Geometry check sheet. Reference: the model listing, model coordinates, mm. Coordinates: 2 decimals unless noted, no trailing zeros. Write each loop counter-clockwise with the first axis right and the second up, starting at its lowest first coordinate (ties: lowest second). Pieces come first, ordered by that corner, then holes. Notation, with made-up numbers: (53.5, 89) -> (110.5, 89) arc R18 ccw to (110.5, 105) -> close; hole circle Ø11 at (30.25, -1). An arc over 180 degrees is marked (long way). Answer in a Markdown table with one row per item. Add a question column.
Q1. Section check C-C, the plane x = 18. Record the boundary of the cut face in (y, z).
Q2. Section check B-B, the plane x = 63. Record the boundary of the cut face in (y, z), and give its area (3 significant figures).
Q3. Section check A-A, the plane z = 0. Record the boundary of the cut face in (x, y).
Q4. Section check D-D, the plane y = 0.9. Record the boundary of the cut face in (x, z).
Q5. Gauge pin test, flat ends, axial feed: P1, Ø3, axis at x = -63.5, z = 23.5, coming from the +Y side; P2, Ø2.5, axis at x = -19, z = -2, coming from the -Y side. Record the tip position at first contact, or that the pin passes through.
Q6. Thickness scan on line 1 (Z direction, x = 63, y = 1.05); line 2 (X direction, y = 4.65, z = 24); line 3 (Z direction, x = 18, y = 2.8). Record the ranges inside material, lowest first.
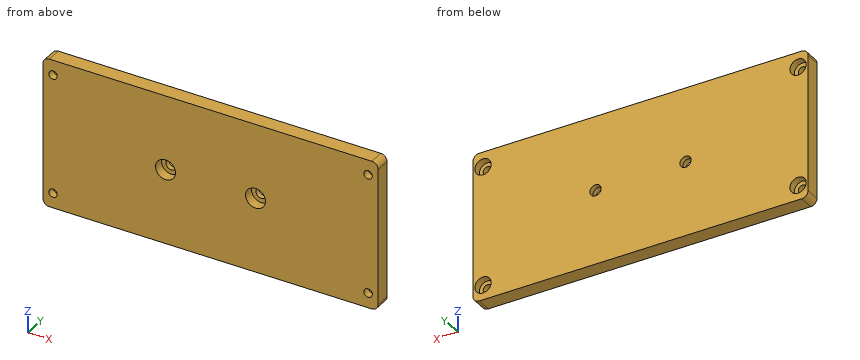
```python
from build123d import *

# Parameters (mm, degrees)
SKETCH1_W                      = 134
SKETCH1_H                      = 60
BOSS_EXTRUDE1_DEPTH            = 6
CBORE_FOR_M3_SHCS1_D           = 3.4
CBORE_FOR_M3_SHCS1_DEPTH       = 17.38
CBORE_FOR_M3_SHCS1_CBORE_D     = 6.5
CBORE_FOR_M3_SHCS1_CBORE_DEPTH = 3
CBORE_FOR_M3_SHCS1_TIP         = 1.021463052
FILLET1_R                      = 2.5
CBORE_FOR_M4_SHCS1_D           = 4.5
CBORE_FOR_M4_SHCS1_DEPTH       = 12
CBORE_FOR_M4_SHCS1_CBORE_D     = 8
CBORE_FOR_M4_SHCS1_CBORE_DEPTH = 4
CBORE_FOR_M4_SHCS1_TIP         = 1.351936393


with BuildPart() as part:
    # Sketch1 → Boss-Extrude1 (new body)
    with BuildSketch(Plane(origin=(0, 0, 0), x_dir=(1, 0, 0), z_dir=(0, 1, 0))):
        Rectangle(SKETCH1_W, SKETCH1_H)
    extrude(amount=BOSS_EXTRUDE1_DEPTH)

    # CBORE for M3 SHCS1
    with Locations(Plane(origin=(0, 6, 0), x_dir=(1, 0, 0), z_dir=(0, 1, 0))):
        with Locations((-63, 24), (-63, -24), (63, -24), (63, 24)):
            CounterBoreHole(CBORE_FOR_M3_SHCS1_D / 2, CBORE_FOR_M3_SHCS1_CBORE_D / 2, CBORE_FOR_M3_SHCS1_CBORE_DEPTH, depth=CBORE_FOR_M3_SHCS1_DEPTH)
            with Locations((0, 0, -(CBORE_FOR_M3_SHCS1_DEPTH + CBORE_FOR_M3_SHCS1_TIP / 2))):  # 118° drill point
                Cone(0, CBORE_FOR_M3_SHCS1_D / 2, CBORE_FOR_M3_SHCS1_TIP, mode=Mode.SUBTRACT)

    # Fillet1
    fillet1_edges = [part.edges().sort_by_distance(p)[0] for p in [
        (67, 3, 30),
        (-67, 3, 30),
        (-67, 3, -30),
        (67, 3, -30),
    ]]
    fillet(fillet1_edges, radius=FILLET1_R)

    # CBORE for M4 SHCS1
    with Locations(Plane.XZ):
        with Locations((-18, 0), (18, 0)):
            CounterBoreHole(CBORE_FOR_M4_SHCS1_D / 2, CBORE_FOR_M4_SHCS1_CBORE_D / 2, CBORE_FOR_M4_SHCS1_CBORE_DEPTH, depth=CBORE_FOR_M4_SHCS1_DEPTH)
            with Locations((0, 0, -(CBORE_FOR_M4_SHCS1_DEPTH + CBORE_FOR_M4_SHCS1_TIP / 2))):  # 118° drill point
                Cone(0, CBORE_FOR_M4_SHCS1_D / 2, CBORE_FOR_M4_SHCS1_TIP, mode=Mode.SUBTRACT)


solid = part.part
```
Calculated:
| question | item | result |
|---|---|---|
| 1 | outline | (0, -30) -> (6, -30) -> (6, -2.25) -> (4, -2.25) -> (4, -4) -> (0, -4) -> close; (0, 4) -> (4, 4) -> (4, 2.25) -> (6, 2.25) -> (6, 30) -> (0, 30) -> close |
| 2 | outline | (0, -30) -> (6, -30) -> (6, -27.25) -> (3, -27.25) -> (3, -25.7) -> (0, -25.7) -> close; (0, -22.3) -> (3, -22.3) -> (3, -20.75) -> (6, -20.75) -> (6, 20.75) -> (3, 20.75) -> (3, 22.3) -> (0, 22.3) -> close; (0, 25.7) -> (3, 25.7) -> (3, 27.25) -> (6, 27.25) -> (6, 30) -> (0, 30) -> close |
| 2 | area | 301 mm² |
| 3 | outline | (-67, 0) -> (-22, 0) -> (-22, 4) -> (-20.25, 4) -> (-20.25, 6) -> (-67, 6) -> close; (-15.75, 4) -> (-14, 4) -> (-14, 0) -> (14, 0) -> (14, 4) -> (15.75, 4) -> (15.75, 6) -> (-15.75, 6) -> close; (20.25, 4) -> (22, 4) -> (22, 0) -> (67, 0) -> (67, 6) -> (20.25, 6) -> close |
| 4 | outline | (-67, -27.5) arc R2.5 ccw to (-64.5, -30) -> (64.5, -30) arc R2.5 ccw to (67, -27.5) -> (67, 27.5) arc R2.5 ccw to (64.5, 30) -> (-64.5, 30) arc R2.5 ccw to (-67, 27.5) -> close; hole circle Ø3.4 at (-63, -24); hole circle Ø3.4 at (-63, 24); hole circle Ø8 at (-18, 0); hole circle Ø8 at (18, 0); hole circle Ø3.4 at (63, -24); hole circle Ø3.4 at (63, 24) |
| 5 | P1 | stops at y = 3 |
| 5 | P2 | stops at y = 4 |
| 6 | line 1 | z = -30 to -25.7, -22.3 to 22.3, 25.7 to 30 |
| 6 | line 2 | x = -67 to -66.25, -59.75 to 59.75, 66.25 to 67 |
| 6 | line 3 | z = -30 to -4, 4 to 30 |
